Could you check a few things on this model? Use its own coordinates, in mm. Face numbers are marked on the shaded views. A direction names the side the tool comes from. Give positions to 0.01 mm unless a question says otherwise; leave off trailing zeros. Write each loop counter-clockwise with the first axis right and the second up, starting at its lowest first coordinate (ties: lowest second). Pieces come first, ordered by that corner, then holes. Notation, with made-up numbers: (-13, -40) - (4, -40) arc R13 ccw to (4, -33) - close; hole circle Ø1 at (47.25, -7). An arc over 180 degrees is marked (long way). Write item = value, one per line.
from build123d import *

# Parameters (mm, degrees)
F1_DEPTH  = 102
F2_R      = 27
F2_R_2    = 18.5
F3_DEPTH  = 30
F4_R      = 10
F5_DEPTH  = 50
F6_R      = 50.99999
F9_DEPTH  = 10
F10_R     = 18.5
F11_DEPTH = 30
F12_R     = 20


# Not quite as in the source:
# - a fillet or chamfer is up to 0.001 mm smaller than in the source, because OpenCascade refuses the exact size


with BuildPart() as f1:
    # F0 (on Top) → F1 (new body)
    with BuildSketch(Plane.XY):
        Polygon((-151.6251202653, -131.7925444834), (-151.6251202653, -156.7925444834), (-27.0366629971, -156.7925444834), (88.4633370029, 43.2593237909), (65.9466765045, 56.2593237909), (-42.6251202653, -131.7925444834), align=None)
    extrude(amount=F1_DEPTH)

    # F2 (on face) → F3 (join)
    with BuildSketch(Plane(origin=(25.099005577, -14.4909176263, 0), x_dir=(-0.5, -0.8660254038, 0), z_dir=(-0.8660254038, 0.5, 0))):
        with Locations((-30.6953418548, 52.0583279431)):
            Circle(F2_R)
        with Locations((-30.6953418548, 52.0583279431)):
            Circle(F2_R_2, mode=Mode.SUBTRACT)
    extrude(amount=F3_DEPTH)

    # F4 (on face) → F5 (cut)
    with BuildSketch(Plane(origin=(0, -131.7925444834, 0), x_dir=(-1, 0, 0), z_dir=(0, 1, 0))):
        with Locations((62.9175528884, 82)):
            Circle(F4_R)
        with Locations((131.9175528884, 82)):
            Circle(F4_R)
        with Locations((131.9175528884, 20)):
            Circle(F4_R)
        with Locations((62.9175528884, 20)):
            Circle(F4_R)
    extrude(amount=-F5_DEPTH, mode=Mode.SUBTRACT)

    # F6 (radius 51 in the source; OpenCascade refuses exactly that, so slightly less here)
    f6_edges = [f1.edges().sort_by_distance(p)[0] for p in [
        (77.205007, 49.759324, 102),
        (77.205007, 49.759324, 0),
    ]]
    fillet(f6_edges, radius=F6_R)

    # F8 (on offset) → F9 (join, symmetric)
    with BuildSketch(Plane(origin=(0, 0, 51), x_dir=(1, 0, 0), z_dir=(0, 0, -1))):
        Polygon((-42.6251202653, 131.7925444834), (-151.6251202653, 131.7925444834), (-4.3144722301, 66.1549466668), align=None)
    extrude(amount=F9_DEPTH, both=True)

    # F10 (on face) → F11 (cut)
    with BuildSketch(Plane(origin=(25.099005577, -14.4909176263, 0), x_dir=(-0.5, -0.8660254038, 0), z_dir=(-0.8660254038, 0.5, 0))):
        with Locations((-30.6953418548, 52.0583279431)):
            Circle(F10_R)
    extrude(amount=-F11_DEPTH, mode=Mode.SUBTRACT)

    # F12
    f12_edges = [f1.edges().sort_by_distance(p)[0] for p in [
        (-151.62512, -144.292544, 102),
        (-151.62512, -144.292544, 0),
    ]]
    fillet(f12_edges, radius=F12_R)


solid = f1.part
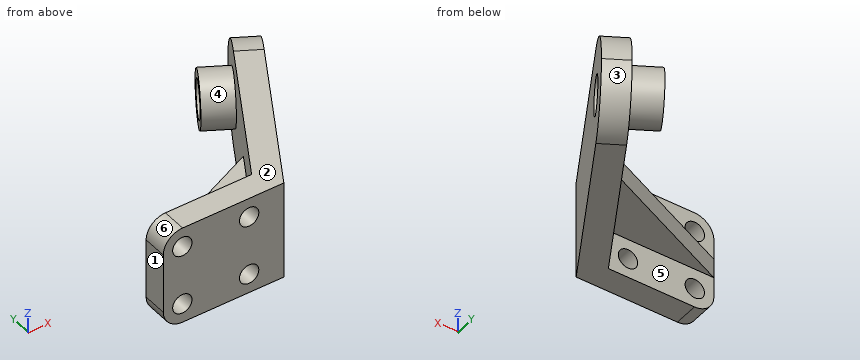
1. If we section it at B-B, the plane x = -93: Please give me the cut outline in (y, z), and give its area (3 significant figures).
Filled sheet:
outline = (-156.79, 0) - (-131.79, 0) - (-131.79, 41) - (-105.67, 41) - (-105.67, 61) - (-131.79, 61) - (-131.79, 102) - (-156.79, 102) - close
area = 3,070 mm2
2. Thinking about a two-plate mould opening in X: for the marked faces 1, 2, 3 and 4, which applies, pulls with the +X half, pulls with the -X half, needs draft (parallel to the pull), parting line crosses it, or undercut?
Filled sheet:
face_1 = pulls with the -X half
face_2 = needs draft
face_3 = pulls with the +X half
face_4 = undercut
3. Which directions (+Z, -Z, +X, -X, +Y, -Y) give clear straight access to the entire face, cutting with the end or side of a thin tool? Please do the marked faces 5 and 6.
Filled sheet:
face_5 = -Z, -X, +Y
face_6 = +Z, -X, +Y, -Y
4. If we section it at A-A, the plane y = -118.5: Please give me the cut outline in (x, z).
Filled sheet:
outline = (-121.79, 41) - (-34.95, 41) - (-34.95, 0) - (-4.93, 0) - (-4.93, 102) - (-34.95, 102) - (-34.95, 61) - (-121.79, 61) - close
5. If we section it at C-C, the plane y = -30: Please give me the cut outline in (x, z), and give its area (3 significant figures).
Filled sheet:
outline = (16.14, 0) - (46.17, 0) - (46.17, 102) - (16.14, 102) - close
area = 3,060 mm2
6. For pin 1 (6 mm diameter, centred on x = 35, z = 74.5, fed in from +Y); pin 2 (3 mm diameter, centred on y = -83.5, z = 71.5, fed in from +X); pin 3 (4 mm diameter, centred on y = 29.5, z = 41.5, fed in from -X); pin 4 (16 mm diameter, centred on x = -131.92, z = 20, fed in from -Y), each with a flat end and sliding along its axis, tell me the tip position at first contact or that it passes through.
Filled sheet:
pin_1 = 37.26
pin_2 = 16.14
pin_3 = 36.05
pin_4 = through
7. I need wall thicknesses on line 1 (Z direction, x = -54, y = -100.5); line 2 (Y direction, x = 30.5, z = 50.5); line 3 (Y direction, x = -81, z = 87). Which ranges of each line are inside material? Lowest first, please.
Filled sheet:
line_1 = 41 to 61
line_2 = -57.14 to -3.45, 39.12 to 48.96
line_3 = -156.79 to -131.79
